Design review of the part built by this model. Coordinates are the model's own, in mm. Face numbers are marked on the shaded views. A direction names the side the tool comes from. Coordinates: 2 decimals unless noted, no trailing zeros. Write each loop counter-clockwise with the first axis right and the second up, starting at its lowest first coordinate (ties: lowest second). Pieces come first, ordered by that corner, then holes.
Q1. The part is to be moulded in two halves that separate along Z. For the marked faces 1, 2 and 3, say which applies: released by +Z, released by -Z, zero draft, split by the parting line, or undercut.
Q2. Take a section at A-A, the plane z = 22.5. Write out the cut boundary in (x, y), plus the area to 3 significant figures.
Q3. For pin 1 Ø8 at (x, y) = (-11.5, -34.5) entering from -Z; pin 2 Ø12 at (x, y) = (-28, -13) entering from -Z; pin 3 Ø3.5 at (x, z) = (0, 22.5) entering from -Y; pin 4 Ø5 at (x, y) = (15.5, -5) entering from -Z, all flat-tipped, find the tip position at first contact; note any pin that passes through.
Q4. Take a section at B-B, the plane x = 0. State how many separate pieces and enclosed holes the cut face has, plus the area to 3 significant figures.
Q5. For L1, parallel to X at y = 1.8, z = -42.5; L2, parallel to Z at x = -4.5, y = -4.5; L3, parallel to X at y = -14, z = -10, list the stretches that pass through material, from the lowest coordinate up.
Q6. Take a section at D-D, the plane z = -10. Write out the cut boundary in (x, y), plus the area to 3 significant figures.
Q7. For the marked faces 4 and 5, list the 3-axis set-ups (+Z, -Z, +X, -X, +Y, -Y) from which the entire face can be reached by the end or side of a thin tool; tool diameter is ignored.
from build123d import *

# Parameters (mm, degrees)
SKETCH1_W           = 105
SKETCH1_H           = 105
BOSS_EXTRUDE1_DEPTH = 3
SKETCH3_R           = 1.15
SKETCH3_R_2         = 2.25
CUT_EXTRUDE1_DEPTH  = 75.306796459
SKETCH4_R           = 8.2
CUT_EXTRUDE2_DEPTH  = 1.6
SKETCH5_R           = 48.5
SKETCH5_R_2         = 45.5
BOSS_EXTRUDE3_DEPTH = 10
SKETCH6_R           = 12.5
CUT_EXTRUDE3_DEPTH  = 75.916620319
BOSS_EXTRUDE4_START = 40.4
SKETCH7_R           = 12.5
BOSS_EXTRUDE4_DEPTH = 40.4
FILLET1_R           = 5
SKETCH8_R           = 2.15
CUT_EXTRUDE4_DEPTH  = 10
SKETCH9_R           = 1.65
CUT_EXTRUDE5_DEPTH  = 82.412898241
FILLET2_R           = 10
SKETCH10_R          = 3.419507724
CUT_EXTRUDE6_DEPTH  = 85.526090694
SKETCH11_W          = 7.1
SKETCH11_H          = 4.6
SKETCH11_W_2        = 4.7
SKETCH11_H_2        = 2.2
BOSS_EXTRUDE5_DEPTH = 5.7
SKETCH12_W          = 7.1
SKETCH12_H          = 4.6
BOSS_EXTRUDE6_DEPTH = 1
SKETCH13_W          = 4.7
SKETCH13_H          = 2.2
CUT_EXTRUDE7_DEPTH  = 3


with BuildPart() as part:
    # Sketch1 → Boss-Extrude1 (new body)
    with BuildSketch(Plane(origin=(0, 0, 0), x_dir=(1, 0, 0), z_dir=(0, 1, 0))):
        Rectangle(SKETCH1_W, SKETCH1_H)
    extrude(amount=BOSS_EXTRUDE1_DEPTH)

    # Sketch3 → Cut-Extrude1 (cut, through all)
    with BuildSketch(Plane(origin=(0, 3, 0), x_dir=(1, 0, 0), z_dir=(0, 1, 0))):
        with Locations(Location((-7.7, -30.2, 0), (0, 0, 270))):
            Circle(SKETCH3_R)
        with Locations(Location((7.7, -30.2, 0), (0, 0, 270))):
            Circle(SKETCH3_R)
        with Locations(Location((7.7, -14.8, 0), (0, 0, 270))):
            Circle(SKETCH3_R)
        with Locations(Location((-7.7, -14.8, 0), (0, 0, 270))):
            Circle(SKETCH3_R)
        with Locations(Location((0, -22.5, 0), (0, 0, 270))):
            Circle(SKETCH3_R_2)
    extrude(amount=-CUT_EXTRUDE1_DEPTH, mode=Mode.SUBTRACT)

    # Sketch4 → Cut-Extrude2 (cut)
    with BuildSketch(Plane(origin=(0, 3, 0), x_dir=(1, 0, 0), z_dir=(0, 1, 0))):
        with Locations(Location((0, -22.5, 0), (0, 0, 270))):
            Circle(SKETCH4_R)
    extrude(amount=-CUT_EXTRUDE2_DEPTH, mode=Mode.SUBTRACT)

    # Sketch5 → Boss-Extrude3 (add)
    with BuildSketch(Plane.XZ):
        with Locations(Location((0, 0, 0), (0, 0, 270))):
            Circle(SKETCH5_R)
        with Locations(Location((0, 0, 0), (0, 0, 270))):
            Circle(SKETCH5_R_2, mode=Mode.SUBTRACT)
    extrude(amount=BOSS_EXTRUDE3_DEPTH)

    # Sketch6 → Cut-Extrude3 (cut, through all)
    with BuildSketch(Plane.XZ):
        with Locations(Location((0, -10, 0), (0, 0, 270))):
            Circle(SKETCH6_R)
    extrude(amount=-CUT_EXTRUDE3_DEPTH, mode=Mode.SUBTRACT)

    # Sketch7 → Boss-Extrude4 (add)
    with BuildSketch(Plane.XZ.offset(BOSS_EXTRUDE4_START)):
        with BuildLine():
            ThreePointArc((-7.60254763, 3.50745237), (-16.035533906, 6.035533906), (-13.50745237, -2.39745237))
            ThreePointArc((-13.50745237, -2.39745237), (-15.5, -10), (-13.50745237, -17.60254763))
            ThreePointArc((-13.50745237, -17.60254763), (-16.035533906, -26.035533906), (-7.60254763, -23.50745237))
            ThreePointArc((-7.60254763, -23.50745237), (0, -25.5), (7.60254763, -23.50745237))
            ThreePointArc((7.60254763, -23.50745237), (16.035533906, -26.035533906), (13.50745237, -17.60254763))
            ThreePointArc((13.50745237, -17.60254763), (15.5, -10), (13.50745237, -2.39745237))
            ThreePointArc((13.50745237, -2.39745237), (16.035533906, 6.035533906), (7.60254763, 3.50745237))
            ThreePointArc((7.60254763, 3.50745237), (0, 5.5), (-7.60254763, 3.50745237))
        make_face()
        with Locations(Location((0, -10, 0), (0, 0, 270))):
            Circle(SKETCH7_R, mode=Mode.SUBTRACT)
    extrude(amount=-BOSS_EXTRUDE4_DEPTH)

    # Fillet1
    fillet1_edges = [part.edges().sort_by_distance(p)[0] for p in [
        (7.60254763, -20.2, 3.50745237),
        (-7.60254763, -20.2, 3.50745237),
        (-13.50745237, -20.2, -2.39745237),
        (-13.50745237, -20.2, -17.60254763),
        (-7.60254763, -20.2, -23.50745237),
        (7.60254763, -20.2, -23.50745237),
        (13.50745237, -20.2, -17.60254763),
        (13.50745237, -20.2, -2.39745237),
    ]]
    fillet(fillet1_edges, radius=FILLET1_R)

    # Sketch8 → Cut-Extrude4 (cut)
    with BuildSketch(Plane.XZ.offset(40.4)):
        with Locations(Location((-12.5, -22.5, 0), (0, 0, 270))):
            Circle(SKETCH8_R)
        with Locations(Location((12.5, -22.5, 0), (0, 0, 270))):
            Circle(SKETCH8_R)
        with Locations(Location((-12.5, 2.5, 0), (0, 0, 270))):
            Circle(SKETCH8_R)
        with Locations(Location((12.5, 2.5, 0), (0, 0, 270))):
            Circle(SKETCH8_R)
    extrude(amount=-CUT_EXTRUDE4_DEPTH, mode=Mode.SUBTRACT)

    # Sketch9 → Cut-Extrude5 (cut, through all)
    with BuildSketch(Plane.XZ.offset(30.4)):
        with Locations(Location((12.5, -22.5, 0), (0, 0, 270))):
            Circle(SKETCH9_R)
        with Locations(Location((-12.5, -22.5, 0), (0, 0, 270))):
            Circle(SKETCH9_R)
        with Locations(Location((-12.5, 2.5, 0), (0, 0, 270))):
            Circle(SKETCH9_R)
        with Locations(Location((12.5, 2.5, 0), (0, 0, 270))):
            Circle(SKETCH9_R)
    extrude(amount=-CUT_EXTRUDE5_DEPTH, mode=Mode.SUBTRACT)

    # Fillet2
    fillet2_edges = [part.edges().sort_by_distance(p)[0] for p in [
        (-52.5, 1.5, -52.5),
        (52.5, 1.5, -52.5),
        (52.5, 1.5, 52.5),
        (-52.5, 1.5, 52.5),
    ]]
    fillet(fillet2_edges, radius=FILLET2_R)

    # Sketch10 → Cut-Extrude6 (cut, through all)
    with BuildSketch(Plane.XZ):
        with Locations(Location((-42.5, -42.5, 0), (0, 0, 270))):
            Circle(SKETCH10_R)
        with Locations(Location((42.5, -42.5, 0), (0, 0, 270))):
            Circle(SKETCH10_R)
        with Locations(Location((42.5, 42.5, 0), (0, 0, 270))):
            Circle(SKETCH10_R)
        with Locations(Location((-42.5, 42.5, 0), (0, 0, 270))):
            Circle(SKETCH10_R)
    extrude(amount=-CUT_EXTRUDE6_DEPTH, mode=Mode.SUBTRACT)

    # Sketch11 → Boss-Extrude5 (add)
    with BuildSketch(Plane.XZ):
        with Locations((0, -31.116528476)):
            Rectangle(SKETCH11_W, SKETCH11_H)
        with Locations((0, -31.116528476)):
            Rectangle(SKETCH11_W_2, SKETCH11_H_2, mode=Mode.SUBTRACT)
    extrude(amount=BOSS_EXTRUDE5_DEPTH)

    # Sketch12 → Boss-Extrude6 (add)
    with BuildSketch(Plane.XZ.offset(5.7)):
        with Locations((0, -31.116528476)):
            Rectangle(SKETCH12_W, SKETCH12_H)
    extrude(amount=BOSS_EXTRUDE6_DEPTH)

    # Sketch13 → Cut-Extrude7 (cut)
    with BuildSketch(Plane.XZ):
        with Locations((0, -31.116528476)):
            Rectangle(SKETCH13_W, SKETCH13_H)
    extrude(amount=-CUT_EXTRUDE7_DEPTH, mode=Mode.SUBTRACT)


solid = part.part
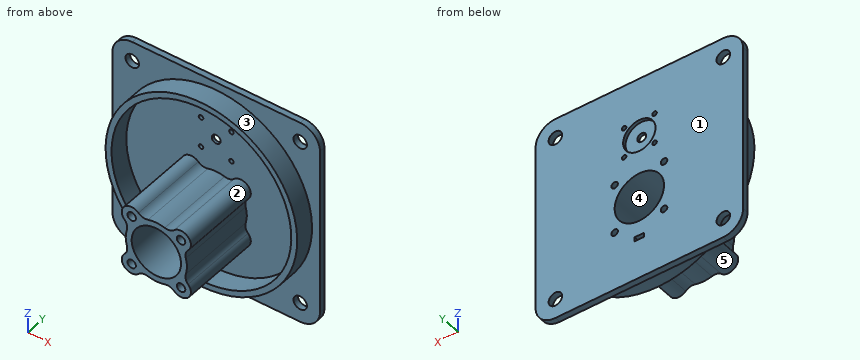
Responses:
1. face 1: zero draft
1. face 2: undercut
1. face 3: split by the parting line
2. outline: (-52.5, 0) - (-42.97, 0) - (-42.97, -10) - (-39.55, -10) - (-39.55, 0) - (-2.25, 0) - (-2.25, 1.4) - (-8.2, 1.4) - (-8.2, 3) - (-52.5, 3) - close; (2.25, 0) - (39.55, 0) - (39.55, -10) - (42.97, -10) - (42.97, 0) - (52.5, 0) - (52.5, 3) - (8.2, 3) - (8.2, 1.4) - (2.25, 1.4) - close
2. area: 351 mm2
3. pin 1: stops at z = -27.5
3. pin 2: stops at z = -42.8
3. pin 3: passes through
3. pin 4: stops at z = -46.73
4. separate pieces: 3
4. enclosed holes: 0
4. area: 522 mm2
5. L1: x = -52.5 to -45.92, -39.08 to 39.08, 45.92 to 52.5
5. L2: z = -48.29 to -45.28, -24.84 to -21.66, 1.66 to 4.84, 45.28 to 48.29
5. L3: x = -15.5 to -12.5, 12.5 to 15.5
6. outline: (-52.5, 0) - (-47.46, 0) - (-47.46, -10) - (-44.39, -10) - (-44.39, 0) - (-15.5, 0) - (-15.5, -40.4) - (-12.5, -40.4) - (-12.5, 3) - (-52.5, 3) - close; (12.5, -40.4) - (15.5, -40.4) - (15.5, 0) - (44.39, 0) - (44.39, -10) - (47.46, -10) - (47.46, 0) - (52.5, 0) - (52.5, 3) - (12.5, 3) - close
6. area: 544 mm2
7. face 4: +Y, -Y
7. face 5: -Y
